Can you work these out from the model? Positions are in its coordinate system, mm. Give positions to 0.01 mm unless a question says otherwise; leave off trailing zeros. Write each loop counter-clockwise with the first axis right and the second up, starting at its lowest first coordinate (ties: lowest second). Pieces come first, ordered by that corner, then holes.
Autodesk Fusion 360 part; units mm, degrees
sketch "Sketch1" plane through (0, 0, 0) normal (0, 0, 1) x (1, 0, 0)
  circle A0 centre (0, 0) radius 3
  circle A1 centre (10, 0) radius 3
  circle A2 centre (20, 0) radius 3
  circle A3 centre (0, 10) radius 3
  circle A4 centre (20, 10) radius 3
  circle A5 centre (10, 10) radius 3
  circle A6 centre (0, 20) radius 3
  circle A7 centre (20, 20) radius 3
  circle A8 centre (10, 20) radius 3
  line L0 (25, 25) -> (-5, 25)
  line L1 (-5, 25) -> (-5, -5)
  line L2 (-5, -5) -> (25, -5)
  line L3 (25, -5) -> (25, 25)
  line L4 (25, 25) -> (-5, -5) construction
  line L5 (-5, 25) -> (25, -5) construction
  point P0 (10, 10)
  dimension "d1" = 6
  dimension "d4" = 20
  dimension "d5" = 0
  dimension "d8" = 0
  dimension "d9" = 20
  dimension "d10" = 30
  dimension "d11" = 30
extrude "Extrude1" add sketch "Sketch1" along normal blind 10
1) If we mould it in two halves opening along Y, with no side actions, what happens to faces 1 (the face through (17.6, 21.8, 4.9)), 2 (the face through (10, -5, 5)), 3 (the face through (25, 10, 5)), 4 (the face through (10, 25, 5))? For each: +Y half, -Y half, draft (parallel to the pull), parting line (faces both ways), or undercut.
Values follow:
face 1: undercut
face 2: -Y half
face 3: draft
face 4: +Y half
2) Suppose I cut it at C-C on z = 8.75. State how many separate pieces and enclosed holes the cut face has, plus the area to 3 significant figures.
Values follow:
separate pieces: 1
enclosed holes: 9
area: 646 mm2
3) For pin 1 Ø5 at (x, y) = (20, 20) entering from -Z, with a flat end and sliding along its axis, tell me the tip position at first contact or that it passes through.
Values follow:
pin 1: passes through
4) Suppose I cut it at A-A on y = 10. Write out the boundary of the cut face in (x, z).
Values follow:
outline: (-5, 0) - (-3, 0) - (-3, 10) - (-5, 10) - close; (3, 0) - (7, 0) - (7, 10) - (3, 10) - close; (13, 0) - (17, 0) - (17, 10) - (13, 10) - close; (23, 0) - (25, 0) - (25, 10) - (23, 10) - close
5) Please list where these lines run through material, in increasing order: L1, parallel to Y at x = 0, z = 4.25; L2, parallel to X at y = 10.5, z = 0.75; L3, parallel to X at y = 12.5, z = 8.
Values follow:
L1: y = -5 to -3, 3 to 7, 13 to 17, 23 to 25
L2: x = -5 to -2.96, 2.96 to 7.04, 12.96 to 17.04, 22.96 to 25
L3: x = -5 to -1.66, 1.66 to 8.34, 11.66 to 18.34, 21.66 to 25
